The model under review builds one solid part; all positions refer to its coordinate system, in mm. Face numbers are marked on the shaded views. Give positions to 0.01 mm unless a question says otherwise; leave off trailing zeros. Loops run counter-clockwise (first coordinate to the right, second up) from the corner with the lowest first, then second, coordinate; pieces in that order, holes last. Notation, with made-up numbers: M 41,-35 L 98,-35 A5 ccw 98,-26 Z; hole C 30,48 d4. An arc over 180 degrees is marked long. Write item = value, one per line. Start each with the question number.
1. We need section A-A on x = -10. Give the boundary of the cut face in (y, z), then the cut area to 3 significant figures.
2. We need section B-B on x = -4.75. Give the boundary of the cut face in (y, z), then the cut area to 3 significant figures.
3. Wall thickness on line 1 along Y through (x, z) = (5.5, 0); line 2 along Z through (x, y) = (5, 4); line 3 along Y through (x, z) = (3.5, 0): over which ranges is each line inside the solid? List them lowest first. Write a range as from..to.
4. Draft analysis for pull direction Y (two halves, no side actions). For the marked faces 1, 2 and 3, state which applies: pulls with the +Y half, pulls with the -Y half, needs draft (parallel to the pull), parting line crosses it, or undercut.
5. For pin 1 (4 mm diameter, centred on y = 8.5, z = -4.5, fed in from -X); pin 2 (1 mm diameter, centred on x = -8, y = 5, fed in from -Z); pin 3 (1.5 mm diameter, centred on x = -11.5, z = -2, fed in from +Y), all flat-tipped, find the tip position at first contact; note any pin that passes through.
from build123d import *

# Parameters (mm, degrees)
SKETCH3_R          = 13.805
CUT_EXTRUDE1_DEPTH = 10
SKETCH4_R          = 5.75
CUT_EXTRUDE2_DEPTH = 11
FILLET1_R          = 0.25


with BuildPart() as part:
    # Sketch1 → Revolve1 (revolve)
    with BuildSketch(Plane(origin=(0, 0, 0), x_dir=(1, 0, 0), z_dir=(0, 1, 0))):
        with BuildLine():
            Line((0, 14), (0, -14))
            ThreePointArc((0, -14), (-14, 0), (0, 14))
        make_face()
    revolve(axis=Axis((0, 0, -14), (0, 0, 1)))

    # Sketch3 → Cut-Extrude1 (cut)
    with BuildSketch(Plane(origin=(9, 0, 0), x_dir=(0, 0, -1), z_dir=(1, 0, 0))):
        Circle(SKETCH3_R)
    extrude(amount=CUT_EXTRUDE1_DEPTH, mode=Mode.SUBTRACT)

    # Sketch4 → Cut-Extrude2 (cut)
    with BuildSketch(Plane(origin=(9, 0, 0), x_dir=(0, 0, -1), z_dir=(1, 0, 0))):
        Circle(SKETCH4_R)
    extrude(amount=-CUT_EXTRUDE2_DEPTH, mode=Mode.SUBTRACT)

    # Sketch6 → Cut-Revolve1 (revolve, cut)
    with BuildSketch(Plane(origin=(0, 0, 0), x_dir=(1, 0, 0), z_dir=(0, 1, 0))):
        Polygon((7, -12.124355653), (9.62, -7.5), (9.62, -12.124355653), align=None)
    revolve(axis=Axis((0, 0, 0), (1, 0, 0)), mode=Mode.SUBTRACT)

    # Fillet1
    fillet1_edges = [part.edges().sort_by_distance(p)[0] for p in [
        (9, 0, 5.75),
        (9, 0, -8.59431317),
        (7, 0, -12.124355653),
    ]]
    fillet(fillet1_edges, radius=FILLET1_R)


solid = part.part
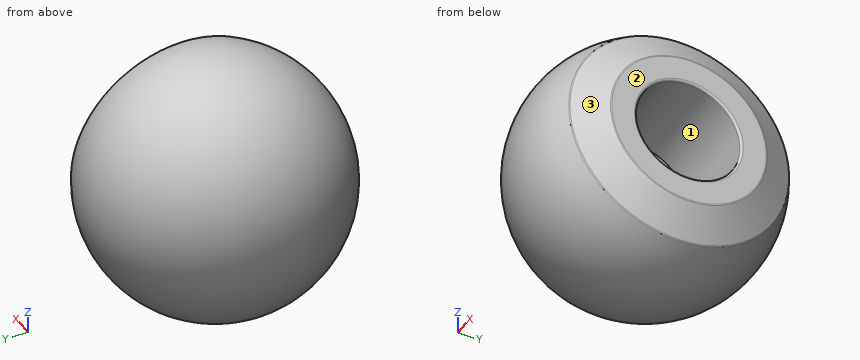
Final values:
q1.outline = C 0,0 d19.6
q1.area = 302 mm²
q2.outline = C 0,0 d26.34
q2.area = 545 mm²
q3.line_1 = -12.87..-5.75, 5.75..12.87
q3.line_2 = -12.45..-4.13, 4.13..12.45
q3.line_3 = -13.56..-5.75, 5.75..13.56
q4.face_1 = undercut
q4.face_2 = needs draft
q4.face_3 = parting line crosses it
q5.pin_1 = -11.75
q5.pin_2 = -10.78
q5.pin_3 = 8.76
